Design review of the part shown in the three views and the two pictorial views. Dimensions are in mm from the part's minimum x, y and z. Round coordinates to 2 decimals unless told otherwise and drop trailing zeros. Loops run counter-clockwise (first coordinate to the right, second up) from the corner with the lowest first, then second, coordinate; pieces in that order, holes last. Notation, with made-up numbers: M 53,54.5 L 75,54.5 A18 cw 75,80.5 Z; hole C 55.5,75 d7. An arc over 180 degrees is marked long. One line per question, with ' | ' between items. Start each with the question number.
1) We need section C-C (y = 9.5). Give the boundary of the cut face in (x, z), and give its area (3 significant figures).
2) For pin 1 Ø0.6 at (y, z) = (0, 0.5) entering from -X, flat-tipped, find the tip position at first contact; note if it passes through.
3) We need section A-A (z = 0.2). Give the boundary of the cut face in (x, y), and give its area (3 significant figures).
4) We need section B-B (x = 1.6). Give the boundary of the cut face in (y, z).
5) For probe 1 along X at (y, z) = (29, 0.5); probe 2 along Y at (x, z) = (2.35, 0.55); probe 3 along Y at (x, z) = (1.4, 0.8), list the stretches that pass through material, from the lowest coordinate up. Write a range as from..to.
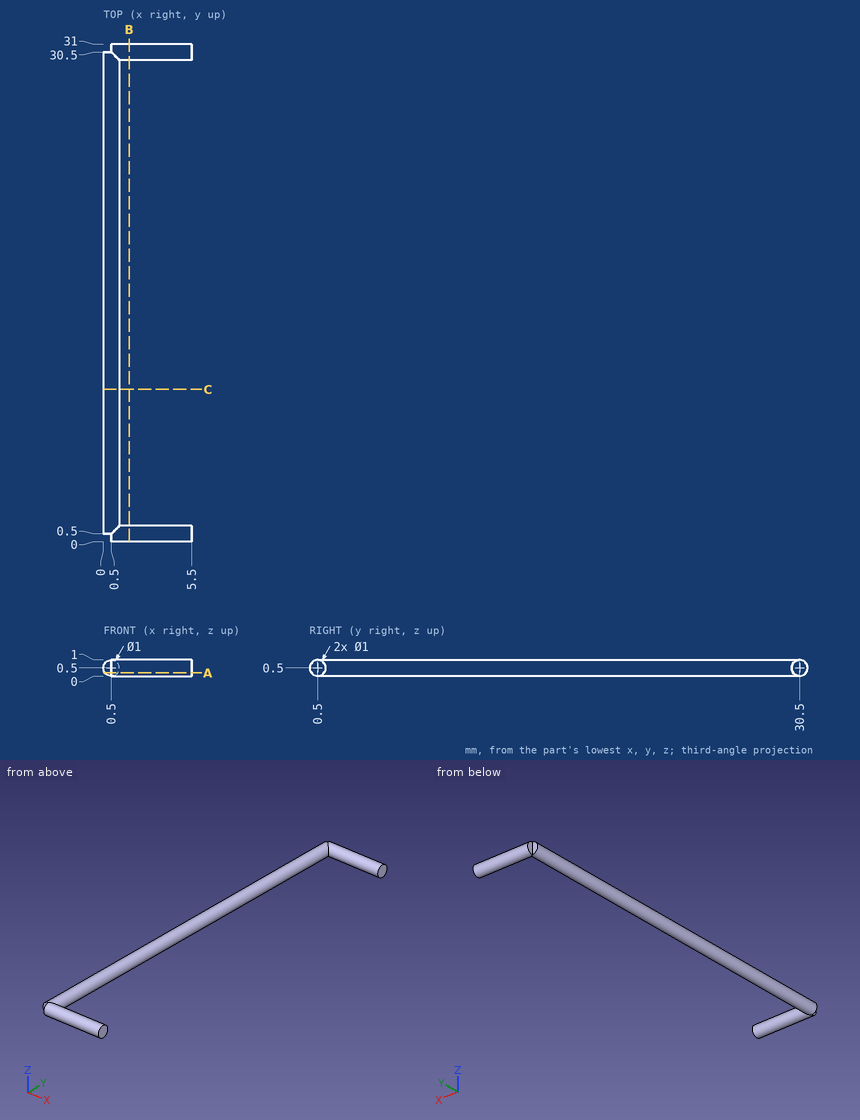
Answers below:
1) outline: C 0.5,0.5 d1 | area: 0.785 mm^2
2) pin 1: x = 0.5
3) outline: M 0.1,0.5 L 0.5,0.5 L 0.5,0.1 L 5.5,0.1 L 5.5,0.9 L 0.9,0.9 L 0.9,30.1 L 5.5,30.1 L 5.5,30.9 L 0.5,30.9 L 0.5,30.5 L 0.1,30.5 Z | area: 31.7 mm^2
4) outline: C 0.5,0.5 d1; C 30.5,0.5 d1
5) probe 1: 0..1 | probe 2: 0..1, 30..31 | probe 3: 0.1..0.9, 30.1..30.9
